Source: CAD feature listing. Evaluate the final solid. Frame: model axes, mm. A direction names the side the tool comes from. Coordinates: 2 decimals unless noted, no trailing zeros. Order: outer loops, then holes, each group sorted by start corner. A loop starts at its lowest first (then second) coordinate and runs counter-clockwise, first axis right, second up. Notation, with made-up numbers: (-12.5, 69) - (13.5, 69) arc R30 cw to (13.5, 91) - close; hole circle Ø8 at (73, 7.5). An arc over 180 degrees is marked (long way). One line per question, with ' | ' between items.
from build123d import *

# Parameters (mm, degrees)
SKETCH2_R           = 1.4224
SKETCH2_R_2         = 0.889
SKETCH2_R_3         = 1.905
BOSS_EXTRUDE1_DEPTH = 2.9718


with BuildPart() as part:
    # Sketch2 → Boss-Extrude1 (new body)
    with BuildSketch(Plane.XY):
        Polygon((0, 6.985), (0, 0), (15.24, 0), (15.24, 28.985), (0, 28.985), (0, 22), (2.9718, 22), (2.9718, 6.985), align=None)
        with Locations((1.4859, 3.4925)):
            Circle(SKETCH2_R, mode=Mode.SUBTRACT)
        with Locations((7.7978, 10.0475)):
            Circle(SKETCH2_R_2, mode=Mode.SUBTRACT)
        with Locations((7.7978, 14.4925)):
            Circle(SKETCH2_R_3, mode=Mode.SUBTRACT)
        with Locations((1.4859, 25.4925)):
            Circle(SKETCH2_R, mode=Mode.SUBTRACT)
        with Locations((7.7978, 18.9375)):
            Circle(SKETCH2_R_2, mode=Mode.SUBTRACT)
    extrude(amount=BOSS_EXTRUDE1_DEPTH)


solid = part.part
(1) Pin query (flat end, axial travel): P1, Ø1.4, axis at x = 7.8, y = 18.94, coming from the -Z side; P2, Ø1.5, axis at y = 17, z = 1, coming from the -X side. Return the tip coordinate at first contact, or that it passes through.
Taken from the geometry:
P1: passes through | P2: stops at x = 2.97
(2) Pull-direction query (X, two-part tool) for faces 1 (the cylindrical face through (0.438, 4.454, 1.465)), 2 (the flat face through (11, 15, 0)), 3 (the flat face through (0, 24.8, 1.5)); classes: pulls with the +X half, pulls with the -X half, needs draft (parallel to the pull), parting line crosses it, or undercut.
Taken from the geometry:
face 1: undercut | face 2: needs draft | face 3: pulls with the -X half
(3) Material intervals for L1, parallel to Y at x = 1.5, z = 1.3 (3 decimals); L2, parallel to Y at x = 7.75, z = 1.05 (3 decimals); L3, parallel to X at y = 20.25, z = 0.9, sorted ascending. Write a range as from..to.
Taken from the geometry:
L1: y = 0..2.07, 4.915..6.985, 22..24.07, 26.915..28.985 | L2: y = 0..9.16, 10.935..12.588, 16.397..18.05, 19.825..28.985 | L3: x = 2.97..15.24
(4) Set-up query: faces 4 (the cylindrical face through (7.68, 19.82, 1.47)), 5 (the flat face through (1, 22, 1)). Return all of +Z, -Z, +X, -X, +Y, -Y with unobstructed straight access to the full face (end or side cutting, diameter ignored); none if empty.
Taken from the geometry:
face 4: +Z, -Z | face 5: +Z, -Z, -X
(5) Cut plane A-A (y = 13.5). Return the cut outline in (x, z).
Taken from the geometry:
outline: (2.97, 0) - (6.17, 0) - (6.17, 2.97) - (2.97, 2.97) - close; (9.42, 0) - (15.24, 0) - (15.24, 2.97) - (9.42, 2.97) - close
(6) Cut plane C-C (z = 0.35). Return the cut outline in (x, y) (1 decimal).
Taken from the geometry:
outline: (0, 0) - (15.2, 0) - (15.2, 29) - (0, 29) - (0, 22) - (3, 22) - (3, 7) - (0, 7) - close; hole circle Ø2.8 at (1.5, 3.5); hole circle Ø2.8 at (1.5, 25.5); hole circle Ø3.8 at (7.8, 14.5); hole circle Ø1.8 at (7.8, 10); hole circle Ø1.8 at (7.8, 18.9)
(7) Cut plane B-B (x = 7.5). Return the cut outline in (y, z) (3 decimals), and give its area (3 significant figures).
Taken from the geometry:
outline: (0, 0) - (9.21, 0) - (9.21, 2.972) - (0, 2.972) - close; (10.885, 0) - (12.611, 0) - (12.611, 2.972) - (10.885, 2.972) - close; (16.374, 0) - (18.1, 0) - (18.1, 2.972) - (16.374, 2.972) - close; (19.775, 0) - (28.985, 0) - (28.985, 2.972) - (19.775, 2.972) - close | area: 65.0 mm²
(8) Cut plane D-D (y = 26.5). Return the cut outline in (x, z), and give its area (3 significant figures).
Taken from the geometry:
outline: (0, 0) - (0.48, 0) - (0.48, 2.97) - (0, 2.97) - close; (2.49, 0) - (15.24, 0) - (15.24, 2.97) - (2.49, 2.97) - close | area: 39.3 mm²
